For this review, use the dimensioned drawing (mm, ordinates from the lowest corner) and the shaded views. A direction names the side the tool comes from. Give positions to 0.01 mm unless a question says otherwise; leave off trailing zeros. Loops run counter-clockwise (first coordinate to the right, second up) from the corner with the lowest first, then second, coordinate; pieces in that order, holes last. Notation, with made-up numbers: (63.25, 72) -> (116.25, 72) arc R25 ccw to (116.25, 96) -> close; hole circle Ø1 at (-20, -36). An arc over 180 degrees is marked (long way). Use a Markdown table: item, result. Add a question column.
1. Add section D-D (x = 13). State the section outline as (y, z) points.
2. For pin 1 Ø2 at (y, z) = (2.5, 2) entering from +X; pin 2 Ø5 at (x, z) = (15, 2.5) entering from +Y; pin 3 Ø3 at (x, z) = (7.5, 6.5) entering from -Y, all flat-tipped, find the tip position at first contact; note any pin that passes through.
3. For the marked faces 1 and 2, list the 3-axis set-ups (+Z, -Z, +X, -X, +Y, -Y) from which the entire face can be reached by the end or side of a thin tool; tool diameter is ignored.
4. Add section B-B (x = 10). State the section outline as (y, z) points, and give its area (3 significant figures).
5. Draft analysis for pull direction Y (two halves, no side actions). For the marked faces 3, 4 and 5, state which applies: pulls with the +Y half, pulls with the -Y half, needs draft (parallel to the pull), parting line crosses it, or undercut.
6. Add section A-A (y = 10). State the section outline as (x, z) points.
7. To check wall thickness, follow line 1 (Y direction, x = 10, z = 1.6); line 2 (Y direction, x = 3.75, z = 2.25); line 3 (Z direction, x = 17, y = 16.5). State the ranges of each line that lie inside material, in increasing order.
8. Add section C-C (z = 4). State the section outline as (x, y) points.
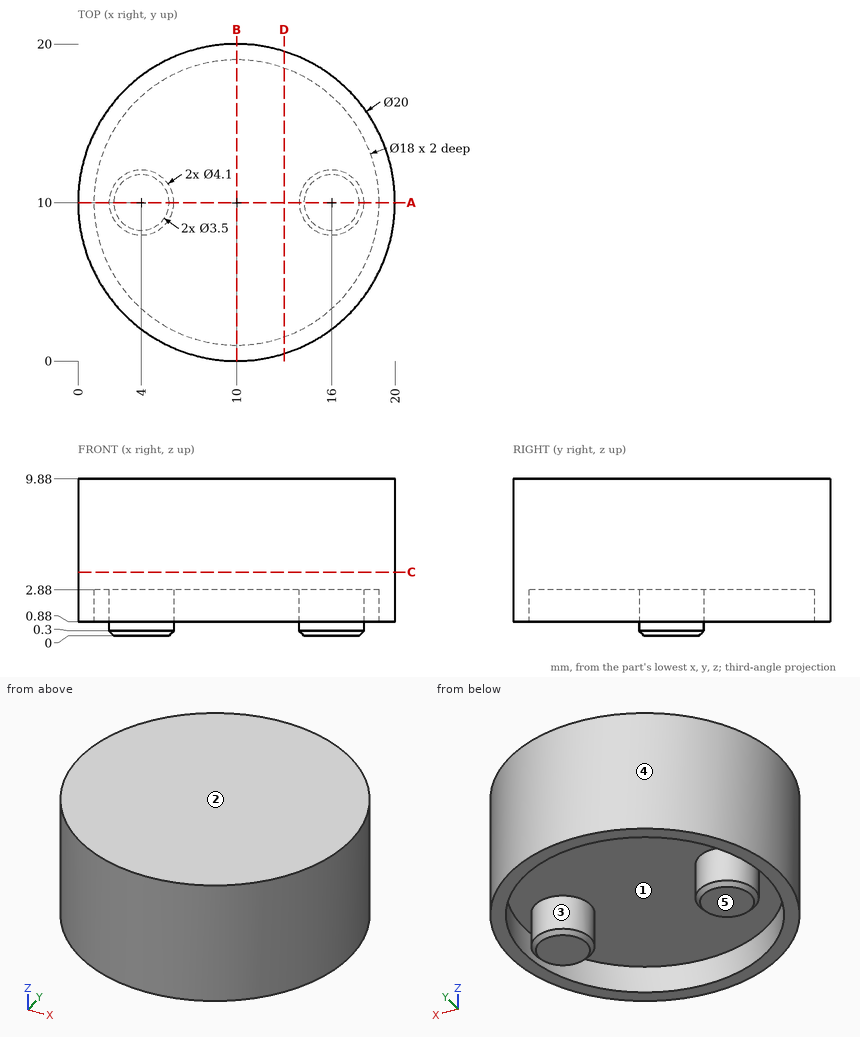
Taken from the geometry:
| question | item | result |
|---|---|---|
| 1 | outline | (0.46, 0.88) -> (1.51, 0.88) -> (1.51, 2.88) -> (18.49, 2.88) -> (18.49, 0.88) -> (19.54, 0.88) -> (19.54, 9.88) -> (0.46, 9.88) -> close |
| 2 | pin 1 | stops at x = 17.6 |
| 2 | pin 2 | stops at y = 19.68 |
| 2 | pin 3 | stops at y = 0.05 |
| 3 | face 1 | -Z |
| 3 | face 2 | +Z, +X, -X, +Y, -Y |
| 4 | outline | (0, 0.88) -> (1, 0.88) -> (1, 2.88) -> (19, 2.88) -> (19, 0.88) -> (20, 0.88) -> (20, 9.88) -> (0, 9.88) -> close |
| 4 | area | 144 mm^2 |
| 5 | face 3 | undercut |
| 5 | face 4 | parting line crosses it |
| 5 | face 5 | needs draft |
| 6 | outline | (0, 0.88) -> (1, 0.88) -> (1, 2.88) -> (1.95, 2.88) -> (1.95, 0.3) -> (2.25, 0) -> (5.75, 0) -> (6.05, 0.3) -> (6.05, 2.88) -> (13.95, 2.88) -> (13.95, 0.3) -> (14.25, 0) -> (17.75, 0) -> (18.05, 0.3) -> (18.05, 2.88) -> (19, 2.88) -> (19, 0.88) -> (20, 0.88) -> (20, 9.88) -> (0, 9.88) -> close |
| 7 | line 1 | y = 0 to 1, 19 to 20 |
| 7 | line 2 | y = 2.19 to 3.52, 7.97 to 12.03, 16.48 to 17.81 |
| 7 | line 3 | z = 0.88 to 9.88 |
| 8 | outline | circle Ø20 at (10, 10) |
